Check sheet for the modelled part. Datum: model origin and axes. Units: mm. A direction names the side the tool comes from. Coordinates: 2 decimals unless noted, no trailing zeros. Order: outer loops, then holes, each group sorted by start corner. A loop starts at its lowest first (then second) coordinate and runs counter-clockwise, first axis right, second up.
1. Cross-section at A-A (x = 0). Enter the section's corners in (y, z).
2. Gauge pin test, flat ends, axial feed: pin 1 Ø1.5 at (y, z) = (-5, 4.5) entering from +X; pin 2 Ø0.5 at (y, z) = (-10.5, 2.5) entering from +X. Record the tip position at first contact, or that the pin passes through.
3. Set-up check for faces 4 (the cylindrical face through (13.4, -9.5, 3)), 5 (the flat face through (13.385, -9.491, 0.493)), 6 (the flat face through (2.075, -6.516, 2.958)), 7 (the flat face through (13.38, -9.5, 5.49)): record each of +Z, -Z, +X, -X, +Y, -Y from which the full face is reachable in a straight line by a thin tool's end or side.
4. Cross-section at C-C (y = -7). Enter the section's corners in (x, z), then the cut area to 3 significant figures.
5. Draft check along Y on faces 1 (the flat face through (13.206, -9.67, 4.746)), 2 (the flat face through (2.7, -6, 0)), 3 (the flat face through (3.14, -6.07, 2.96)). Enter one of: released by +Y, released by -Y, zero draft, split by the parting line, or undercut.
6. Thickness scan on line 1 (Y direction, x = 0, z = 3.45); line 2 (X direction, y = -16.75, z = 1.5); line 3 (X direction, y = -1.5, z = 1). Record the ranges inside material, lowest first.
7. Cross-section at B-B (z = 3.25). Count the separate pieces of the cut face and the enclosed holes in it, then the cut area to 3 significant figures.
```python
from build123d import *

# Parameters (mm, degrees)
EXTRUDE_1_DEPTH          = 6
EXTRUDE_START            = -3.991967
EXTRUDE_2_DEPTH          = 3.991967
PATTERN_CIRCULAR_1_COUNT = 2
PATTERN_CIRCULAR_1_ANGLE = 45
SKETCH_4_R               = 3
CUT_EXTRUDE_2_DEPTH      = 7.0000001


with BuildPart() as part:
    # Sketch 1 → Extrude 1 (new body)
    with BuildSketch(Plane.XY):
        with BuildLine():
            Line((-4.5, 0), (-4.5, -18.2))
            Line((-4.5, -18.2), (-3, -18.2))
            Line((-3, -18.2), (-3, -14.6))
            ThreePointArc((-3, -14.6), (-1.968245837, -12.85), (-3, -11.1))
            Line((-3, -11.1), (-3, -10))
            Line((-3, -10), (3, -10))
            Line((3, -10), (3, -11.1))
            ThreePointArc((3, -11.1), (1.968245837, -12.85), (3, -14.6))
            Line((3, -14.6), (3, -18.2))
            Line((3, -18.2), (4.5, -18.2))
            Line((4.5, -18.2), (4.5, 0))
            ThreePointArc((4.5, 0), (0, 4.5), (-4.5, 0))
        make_face()
    extrude_1 = extrude(amount=EXTRUDE_1_DEPTH)

    # Sketch 3 → Extrude 2 (add)
    with BuildSketch(Plane.XZ.offset(18.2).offset(EXTRUDE_START)):
        with BuildLine():
            Line((-3, 6), (-3, 0))
            Line((-3, 0), (-2.5, 1))
            Line((-2.5, 1), (-2.5, 1.5))
            ThreePointArc((-2.5, 1.5), (-2.757359313, 3), (-2.5, 4.5))
            Line((-2.5, 4.5), (-2.5, 5))
            Line((-2.5, 5), (-3, 6))
        make_face()
        with BuildLine():
            Line((3, 0), (2.5, 1))
            Line((2.5, 1), (2.5, 1.5))
            ThreePointArc((2.5, 1.5), (2.757359313, 3), (2.5, 4.5))
            Line((2.5, 4.5), (2.5, 5))
            Line((2.5, 5), (3, 6))
            Line((3, 6), (3, 0))
        make_face()
    extrude_2 = extrude(amount=EXTRUDE_2_DEPTH)

    # Pattern Circular 1: Extrude 1, Extrude 2 ×2 about axis
    pattern_circular_1_axis = Axis((0, 0, 0), (0, 0, 1))
    for i in range(1, PATTERN_CIRCULAR_1_COUNT):
        add(extrude_1.rotate(pattern_circular_1_axis, i * PATTERN_CIRCULAR_1_ANGLE / (PATTERN_CIRCULAR_1_COUNT - 1)))
        add(extrude_2.rotate(pattern_circular_1_axis, i * PATTERN_CIRCULAR_1_ANGLE / (PATTERN_CIRCULAR_1_COUNT - 1)))

    # Sketch 4 → Cut-Extrude 2 (cut, through all)
    with BuildSketch(Plane(origin=(0, 0, 0), x_dir=(-1, 0, 0), z_dir=(0, 0, -1))):
        Circle(SKETCH_4_R)
        with BuildLine():
            Line((3, -8.75), (3, -3.354101966))
            ThreePointArc((3, -3.354101966), (1.038095674, -4.378625055), (-1.174936357, -4.343906601))
            Line((-1.174936357, -4.343906601), (-3, -8.75))
            Line((-3, -8.75), (3, -8.75))
        make_face()
        with BuildLine():
            Line((-8.308504679, -4.065863992), (-4.493028589, -0.250387902))
            ThreePointArc((-4.493028589, -0.250387902), (-3.830199959, -2.362110978), (-2.240800349, -3.90241128))
            Line((-2.240800349, -3.90241128), (-4.065863992, -8.308504679))
            Line((-4.065863992, -8.308504679), (-8.308504679, -4.065863992))
        make_face()
    extrude(amount=-CUT_EXTRUDE_2_DEPTH, mode=Mode.SUBTRACT)


solid = part.part
```
Data:
1. outline: (-10, 0) - (-8.75, 0) - (-8.75, 6) - (-10, 6) - close; (-4.5, 0) - (-3, 0) - (-3, 6) - (-4.5, 6) - close; (3, 0) - (4.5, 0) - (4.5, 6) - (3, 6) - close
2. pin 1: stops at x = 12.11
2. pin 2: stops at x = 15.49
3. face 4: -Y
3. face 5: -Z, -Y
3. face 6: +Z, -Z
3. face 7: +Z, -Y
4. outline: (-4.5, 0) - (-3, 0) - (-3, 6) - (-4.5, 6) - close; (2.28, 0) - (3.52, 0) - (3.52, 6) - (2.28, 6) - close; (5.37, 0) - (7.14, 0) - (7.14, 6) - (5.37, 6) - close; (10.03, 0) - (13.36, 0) - (13.36, 6) - (10.03, 6) - close
4. area: 47.1 mm2
5. face 1: released by -Y
5. face 2: zero draft
5. face 3: undercut
6. line 1: y = -10 to -8.75, -4.5 to -3, 3 to 4.5
6. line 2: x = -4.5 to -2.5, 2.5 to 4.5
6. line 3: x = -4.5 to -2.6, 2.6 to 4.24, 5.74 to 7.86
7. separate pieces: 1
7. enclosed holes: 3
7. area: 144 mm2
